The figure shows three views and two pictorial views of one solid part (mm, origin at its lowest corner). Answer the questions. A direction names the side the tool comes from. Coordinates: 2 decimals unless noted, no trailing zeros. Order: outer loops, then holes, each group sorted by start corner. A loop starts at its lowest first (then second) coordinate and runs counter-clockwise, first axis right, second up. Notation, with made-up numbers: (32, -24) -> (48, -24) arc R24 ccw to (48, 7) -> close; hole circle Ø6 at (35, 19). An arc over 180 degrees is marked (long way). Return JSON: item names as keys, results as strings.
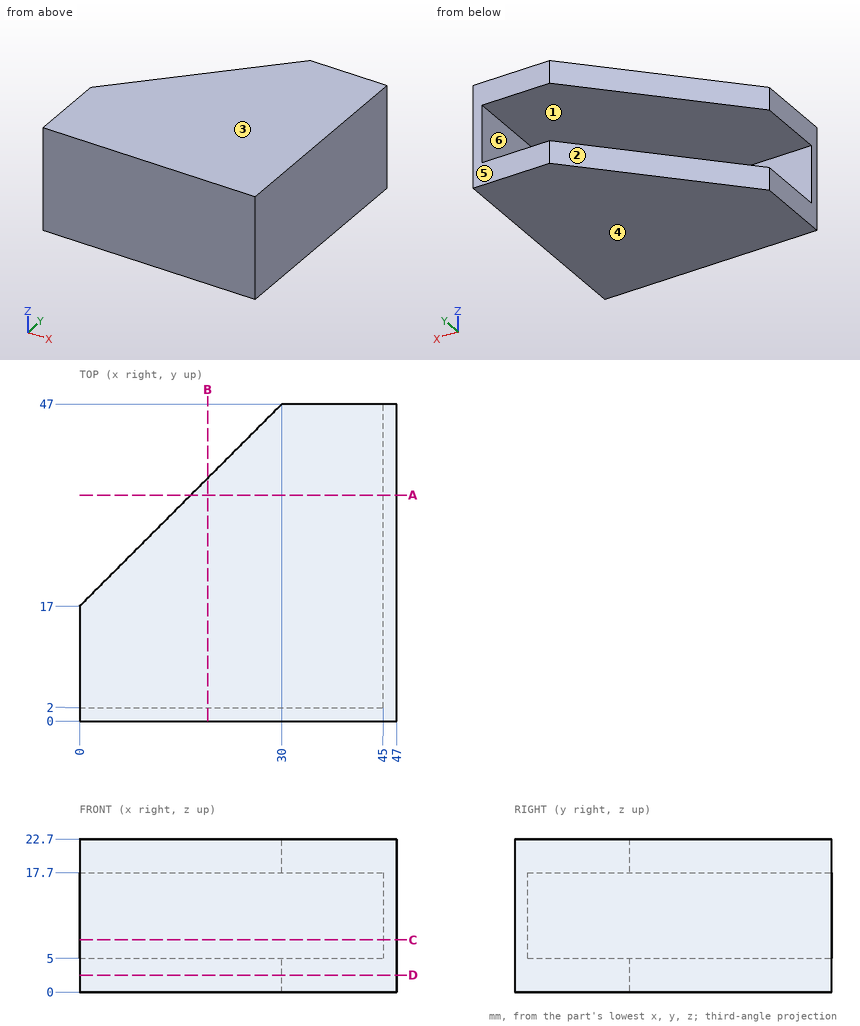
Item 1: Find the intervals of material crossed by probe 1 along Z at (x, y) = (30, 25); probe 2 along X at (y, z) = (7, 9.5); probe 3 along Y at (x, z) = (31, 6.5), in increasing order.
Answer list:
{"probe 1": "0 to 5, 17.7 to 22.7", "probe 2": "45 to 47", "probe 3": "0 to 2"}
Item 2: The part is cut by section A-A on y = 33.5. Determine the outline of the cut face in (x, z).
Answer list:
{"outline": "(16.5, 0) -> (47, 0) -> (47, 22.7) -> (16.5, 22.7) -> (16.5, 17.7) -> (45, 17.7) -> (45, 5) -> (16.5, 5) -> close"}
Item 3: The part is cut by section B-B on x = 19. Determine the outline of the cut face in (y, z).
Answer list:
{"outline": "(0, 0) -> (36, 0) -> (36, 5) -> (2, 5) -> (2, 17.7) -> (36, 17.7) -> (36, 22.7) -> (0, 22.7) -> close"}
Item 4: The part is cut by section D-D on z = 2.5. Determine the outline of the cut face in (x, y).
Answer list:
{"outline": "(0, 0) -> (47, 0) -> (47, 47) -> (30, 47) -> (0, 17) -> close"}
Item 5: Determine the mould class of the marked faces 1, 2, 3 and 4 for opening direction Z: pulls with the +Z half, pulls with the -Z half, needs draft (parallel to the pull), parting line crosses it, or undercut.
Answer list:
{"face 1": "undercut", "face 2": "needs draft", "face 3": "pulls with the +Z half", "face 4": "pulls with the -Z half"}
Item 6: The part is cut by section C-C on z = 7.75. Determine the outline of the cut face in (x, y), plus the area to 3 significant figures.
Answer list:
{"outline": "(0, 0) -> (47, 0) -> (47, 47) -> (45, 47) -> (45, 2) -> (0, 2) -> close", "area": "184 mm2"}
Item 7: Which of the six approach directions +Z, -Z, +X, -X, +Y, -Y give full straight-line access (tool end or side, diameter ignored) to the marked faces 5 and 6?
Answer list:
{"face 5": "+Z, -Z, +X, -X, +Y", "face 6": "-X, +Y"}
Item 8: Flat-ended cylindrical pins translate along their axes: pin 1 (4 mm diameter, centred on y = 21.5, z = 5.5, fed in from -X); pin 2 (6.5 mm diameter, centred on y = 14, z = 12, fed in from -X); pin 3 (3 mm diameter, centred on x = 15, z = 12, fed in from +Y). Find the tip coordinate at first contact, or state that the pin passes through.
Answer list:
{"pin 1": "x = 2.56", "pin 2": "x = 45", "pin 3": "y = 2"}
